Could you check a few things on this model? Use its own coordinates, in mm. A direction names the side the tool comes from. Round coordinates to 2 decimals unless told otherwise and drop trailing zeros. Loops run counter-clockwise (first coordinate to the right, second up) from the corner with the lowest first, then second, coordinate; pieces in that order, holes last. Notation, with made-up numbers: (62.25, -23) -> (121.25, -23) arc R19 ccw to (121.25, 4) -> close; hole circle Ø5 at (74.25, 21). An arc over 180 degrees is marked (long way). One line per item, written item: value.
Autodesk Inventor part; units mm, degrees
ref_plane "YZ Plane" through (0, 0, 0) normal (1, 0, 0) x (0, 1, 0)
ref_plane "XZ Plane" through (0, 0, 0) normal (0, 1, 0) x (-1, 0, 0)
ref_plane "XY Plane" through (0, 0, 0) normal (0, 0, 1) x (1, 0, 0)
sketch "Sketch1" plane through (0, 0, 0) normal (0, 0, 1) x (1, 0, 0)
  line L0 (-40, -21.15) -> (40, -21.15)
  line L1 (40, -21.15) -> (40, 21.15)
  line L2 (40, 21.15) -> (-40, 21.15)
  line L3 (-40, 21.15) -> (-40, -21.15)
  line L4 (-15.5, -15.5) -> (15.5, -15.5) construction
  line L5 (15.5, -15.5) -> (15.5, 15.5) construction
  line L6 (15.5, 15.5) -> (-15.5, 15.5) construction
  line L7 (-15.5, 15.5) -> (-15.5, -15.5) construction
  line L8 (-15.5, -15.5) -> (15.5, 15.5) construction
  line L9 (15.5, -15.5) -> (-15.5, 15.5) construction
  circle A0 centre (-15.5, 15.5) radius 2
  circle A1 centre (15.5, 15.5) radius 2
  circle A2 centre (15.5, -15.5) radius 2
  circle A3 centre (-15.5, -15.5) radius 2
  circle A4 centre (-35, 15.5) radius 1.5
  circle A5 centre (-35, -15.5) radius 1.5
  circle A6 centre (35, -15.5) radius 1.5
  circle A7 centre (35, 15.5) radius 1.5
  circle A8 centre (0, 0) radius 11.5
  point P0 (-40, 0)
  point P1 (0, 21.15)
  dimension "d0" = 80
  dimension "d1" = 42.3
  dimension "d2" = 31
  dimension "d3" = 31
  dimension "d4" = 4
  dimension "d5" = 4
  dimension "d6" = 4
  dimension "d7" = 4
  dimension "d8" = 3
  dimension "d9" = 3
  dimension "d10" = 3
  dimension "d11" = 3
  dimension "d12" = 5
  dimension "d13" = 5
  dimension "d17" = 23
extrude "Extrusion1" add sketch "Sketch1" along normal mid plane 3
fillet "Fillet1" radius 2 4 edges at (-40, -21.15, 0) (-40, 21.15, 0) (40, -21.15, 0) (40, 21.15, 0)
sketch "Sketch2" plane through (0, 0, 1.5) normal (0, 0, 1) x (1, 0, 0)
  arc A0 (40, 19.15) -> (38, 21.15) centre (38, 19.15) ccw
  line L0 (38, 21.15) -> (-38, 21.15)
  arc A1 (-38, 21.15) -> (-40, 19.15) centre (-38, 19.15) ccw
  line L1 (-40, 19.15) -> (-40, -19.15)
  arc A2 (-40, -19.15) -> (-38, -21.15) centre (-38, -19.15) ccw
  line L2 (-38, -21.15) -> (38, -21.15)
  arc A3 (38, -21.15) -> (40, -19.15) centre (38, -19.15) ccw
  line L3 (40, -19.15) -> (40, 19.15)
  circle A4 centre (0, 0) radius 11.5
  circle A5 centre (-15.5, 15.5) radius 2
  circle A6 centre (15.5, 15.5) radius 2
  circle A7 centre (15.5, -15.5) radius 2
  circle A8 centre (-15.5, -15.5) radius 2
  circle A9 centre (-35, 15.5) radius 1.5
  circle A10 centre (-35, -15.5) radius 1.5
  circle A11 centre (35, -15.5) radius 1.5
  circle A12 centre (35, 15.5) radius 1.5
  line L4 (-38, -21.15) -> (38, -21.15)
  line L5 (-28, -21.15) -> (28, -21.15)
  line L6 (28, -21.15) -> (28, 21.15)
  line L7 (28, 21.15) -> (-28, 21.15)
  line L8 (-28, 21.15) -> (-28, -21.15)
  point P0 (-28, 21.15)
  dimension "d18" = 12
  dimension "d19" = 12
extrude "Extrusion2" add sketch "Sketch2" along normal blind 5.3 contours L3 A3 L2 L6 L0 A0 | L8 L2 A2 L1 A1 L0
properties part number "3217a_Stepper Motor Plate_V1" material "Aluminum 6061"
(1) We'd pull the mould along Y, two halves only. Please class faces 1 (the face through (-39.43, 20.55, 2.59)), 2 (the face through (-39.43, -20.55, 2.71)), 3 (the face through (-15.76, -17.483, -0.021)): +Y half, -Y half, draft (parallel to the pull), parting line (faces both ways), or undercut.
Results below:
face 1: +Y half
face 2: -Y half
face 3: undercut
(2) Imagine slicing it at B-B on y = 15.5. Write out the boundary of the cut face in (x, z).
Results below:
outline: (-40, -1.5) -> (-36.5, -1.5) -> (-36.5, 6.8) -> (-40, 6.8) -> close; (-33.5, -1.5) -> (-17.5, -1.5) -> (-17.5, 1.5) -> (-28, 1.5) -> (-28, 6.8) -> (-33.5, 6.8) -> close; (-13.5, -1.5) -> (13.5, -1.5) -> (13.5, 1.5) -> (-13.5, 1.5) -> close; (17.5, -1.5) -> (33.5, -1.5) -> (33.5, 6.8) -> (28, 6.8) -> (28, 1.5) -> (17.5, 1.5) -> close; (36.5, -1.5) -> (40, -1.5) -> (40, 6.8) -> (36.5, 6.8) -> close
(3) Imagine slicing it at C-C on x = -15.5. Write out the boundary of the cut face in (y, z), then the cut area to 3 significant figures.
Results below:
outline: (-21.15, -1.5) -> (-17.5, -1.5) -> (-17.5, 1.5) -> (-21.15, 1.5) -> close; (-13.5, -1.5) -> (13.5, -1.5) -> (13.5, 1.5) -> (-13.5, 1.5) -> close; (17.5, -1.5) -> (21.15, -1.5) -> (21.15, 1.5) -> (17.5, 1.5) -> close
area: 103 mm²
(4) Please list where these lines run through material, in increasing order: L1, parallel to Y at x = -15.5, z = 0.05; L2, parallel to Y at x = 35, z = 3.25; L3, parallel to X at y = -10.5, z = 3.5.
Results below:
L1: y = -21.15 to -17.5, -13.5 to 13.5, 17.5 to 21.15
L2: y = -21.15 to -17, -14 to 14, 17 to 21.15
L3: x = -40 to -28, 28 to 40
(5) Imagine slicing it at A-A on z = 5.75. Write out the boundary of the cut face in (x, y).
Results below:
outline: (-40, -19.15) arc R2 ccw to (-38, -21.15) -> (-28, -21.15) -> (-28, 21.15) -> (-38, 21.15) arc R2 ccw to (-40, 19.15) -> close; (28, -21.15) -> (38, -21.15) arc R2 ccw to (40, -19.15) -> (40, 19.15) arc R2 ccw to (38, 21.15) -> (28, 21.15) -> close; hole circle Ø3 at (-35, -15.5); hole circle Ø3 at (-35, 15.5); hole circle Ø3 at (35, -15.5); hole circle Ø3 at (35, 15.5)
(6) For pin 1 Ø1.5 at (x, y) = (20.5, 1.5) entering from +Z; pin 2 Ø2.5 at (x, y) = (-35, 15.5) entering from -Z, each with a flat end and sliding along its axis, tell me the tip position at first contact or that it passes through.
Results below:
pin 1: stops at z = 1.5
pin 2: passes through
(7) On a 3-axis mill with a long thin cutter (end or side, diameter ignored), from which of +Z, -Z, +X, -X, +Y, -Y can I reach the whole of each face in a straight line? I mean faces 4 (the face through (-9, -9, -1.5)), 5 (the face through (-7, 10, 1.5)). Say none if no direction works.
Results below:
face 4: -Z, +X, -X, +Y, -Y
face 5: +Z, +Y, -Y
(8) Imagine slicing it at D-D on x = 0. Write out the boundary of the cut face in (y, z).
Results below:
outline: (-21.15, -1.5) -> (-11.5, -1.5) -> (-11.5, 1.5) -> (-21.15, 1.5) -> close; (11.5, -1.5) -> (21.15, -1.5) -> (21.15, 1.5) -> (11.5, 1.5) -> close
